Verification items for this drawing (mm, ordinates from the low corner). A direction names the side the tool comes from. Round coordinates to 2 decimals unless told otherwise and drop trailing zeros. Write each loop counter-clockwise with the first axis right and the second up, starting at its lowest first coordinate (ties: lowest second). Pieces come first, ordered by that corner, then holes. Notation, with made-up numbers: (81, -27.75) -> (94, -27.75) arc R28 ccw to (94, -8.75) -> close; hole circle Ø6 at (4, -1.5). An arc over 180 degrees is marked (long way). Put each result on its own line as item: value. Start each with the question number.
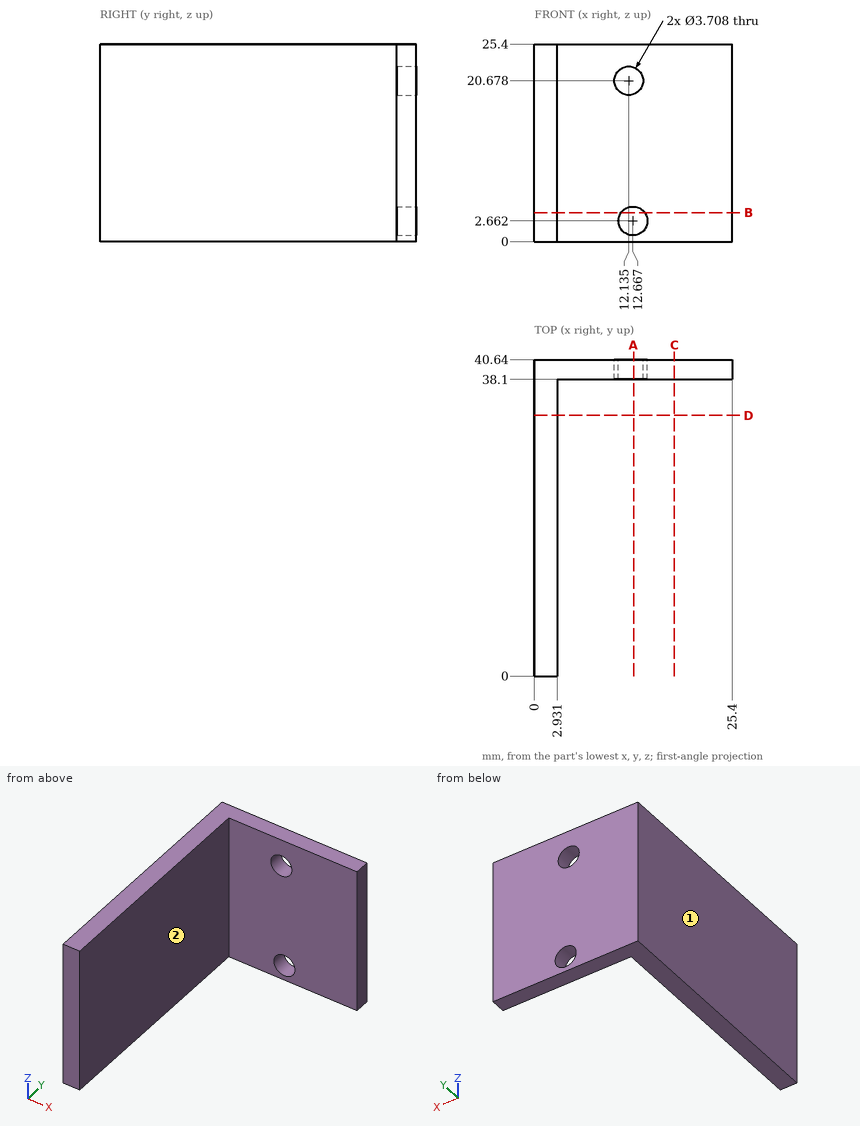
1. Gauge pin test, flat ends, axial feed: P1, Ø5, axis at y = 31, z = 4.5, coming from the +X side; P2, Ø11, axis at x = 9.5, z = 12.5, coming from the -Y side. Record the tip position at first contact, or that the pin passes through.
2. Section check B-B, the plane z = 3.75. Enter the section's corners in (x, y).
3. Section check D-D, the plane y = 33.5. Enter the section's corners in (x, z).
4. Material ranges on L1, parallel to Y at x = 9.25, z = 5.75; L2, parallel to X at y = 11, z = 10.5; L3, parallel to X at y = 38.5, z = 21.75, recorded low to high. Write a range as [from, to].
5. Section check C-C, the plane x = 18. Enter the section's corners in (y, z).
6. Access from +Z, -Z, +X, -X, +Y, -Y to the whole of each face (thin tool, end or side, straight path). Record for the marked faces 1 and 2.
7. Section check A-A, the plane x = 12.75. Enter the section's corners in (y, z) (1 decimal).
Reply:
1. P1: stops at x = 2.93
1. P2: stops at y = 38.1
2. outline: (0, 0) -> (2.93, 0) -> (2.93, 38.1) -> (11.17, 38.1) -> (11.17, 40.64) -> (0, 40.64) -> close; (14.17, 38.1) -> (25.4, 38.1) -> (25.4, 40.64) -> (14.17, 40.64) -> close
3. outline: (0, 0) -> (2.93, 0) -> (2.93, 25.4) -> (0, 25.4) -> close
4. L1: y = [38.1, 40.64]
4. L2: x = [0, 2.93]
4. L3: x = [0, 10.62], [13.65, 25.4]
5. outline: (38.1, 0) -> (40.64, 0) -> (40.64, 25.4) -> (38.1, 25.4) -> close
6. face 1: +Z, -Z, -X, +Y, -Y
6. face 2: +Z, -Z, +X, -Y
7. outline: (38.1, 0) -> (40.6, 0) -> (40.6, 0.8) -> (38.1, 0.8) -> close; (38.1, 4.5) -> (40.6, 4.5) -> (40.6, 18.9) -> (38.1, 18.9) -> close; (38.1, 22.4) -> (40.6, 22.4) -> (40.6, 25.4) -> (38.1, 25.4) -> close
